from build123d import *

# Parameters (mm, degrees)
SKETCH_1_W          = 132
SKETCH_1_H          = 400
EXTRUDE_1_DEPTH     = 10
SKETCH_2_W          = 23
SKETCH_2_H          = 400
EXTRUDE_2_DEPTH     = 5
SKETCH_3_W          = 16
SKETCH_3_H          = 400
EXTRUDE_3_DEPTH     = 1
SKETCH_4_W          = 20
SKETCH_4_H          = 20
CUT_EXTRUDE_1_DEPTH = 11


with BuildPart() as part:
    # ｽｹｯﾁ1 → ﾎﾞｽ - 押し出し1 (new body)
    with BuildSketch(Plane.XY):
        with Locations((66, 200)):
            Rectangle(SKETCH_1_W, SKETCH_1_H)
    extrude(amount=EXTRUDE_1_DEPTH)

    # ｽｹｯﾁ2 → ﾎﾞｽ - 押し出し2 (add)
    with BuildSketch(Plane.XY.offset(10)):
        with Locations((11.5, 200)):
            Rectangle(SKETCH_2_W, SKETCH_2_H)
    extrude(amount=EXTRUDE_2_DEPTH)

    # ｽｹｯﾁ3 → ﾎﾞｽ - 押し出し3 (add)
    with BuildSketch(Plane.XY.offset(10)):
        with Locations((124, 200)):
            Rectangle(SKETCH_3_W, SKETCH_3_H)
    extrude(amount=EXTRUDE_3_DEPTH)

    # ｽｹｯﾁ4 → ｶｯﾄ - 押し出し1 (cut, through all)
    with BuildSketch(Plane.XY.offset(10)):
        with Locations((77.75, 200)):
            Rectangle(SKETCH_4_W, SKETCH_4_H)
    extrude(amount=-CUT_EXTRUDE_1_DEPTH, mode=Mode.SUBTRACT)


solid = part.part
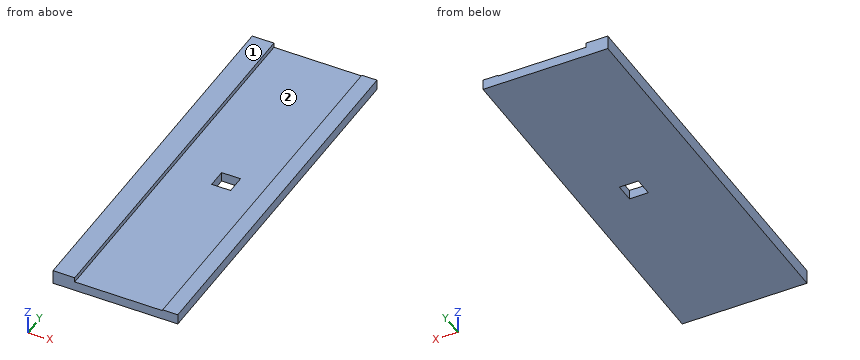
Here's how the part is built. I have some questions about the finished solid (model axes, mm). Face numbers are marked on the shaded views. Coordinates: 2 decimals unless noted, no trailing zeros. Write each loop counter-clockwise with the first axis right and the second up, starting at its lowest first coordinate (ties: lowest second). Pieces come first, ordered by that corner, then holes. Notation, with made-up numbers: (24, -1) - (39, -1) arc R16 ccw to (39, 26) - close; hole circle Ø3 at (-33, 86.5). An arc over 180 degrees is marked (long way). Use one line per item in the form item = value.
1) Suppose I cut it at A-A, the plane x = 73. Write out the boundary of the cut face in (y, z), plus the area to 3 significant figures.
Solved:
outline = (0, 0) - (190, 0) - (190, 10) - (0, 10) - close; (210, 0) - (400, 0) - (400, 10) - (210, 10) - close
area = 3,800 mm2
2) Thinking about a two-plate mould opening in X: for the marked faces 1 and 2, which applies, released by +X, released by -X, zero draft, split by the parting line, or undercut?
Solved:
face_1 = zero draft
face_2 = undercut
3) I need wall thicknesses on line 1 (Y direction, x = 73.5, z = 1.75); line 2 (X direction, y = 86, z = 10.75); line 3 (X direction, y = 104.5, z = 12). Which ranges of each line are inside material? Lowest first, please.
Solved:
line_1 = 0 to 190, 210 to 400
line_2 = 0 to 23, 116 to 132
line_3 = 0 to 23
4) Suppose I cut it at B-B, the plane y = 39.5. Write out the boundary of the cut face in (x, z), plus the area to 3 significant figures.
Solved:
outline = (0, 0) - (132, 0) - (132, 11) - (116, 11) - (116, 10) - (23, 10) - (23, 15) - (0, 15) - close
area = 1,450 mm2
5) I'm going to push flat-ended pins straight in: P1, Ø1, axis at x = 70, y = 354.5, coming from the +Z side; P2, Ø13, axis at x = 124.5, y = 150, coming from the +Z side. Where does each tip first touch, or does it pass through?
Solved:
P1 = 10
P2 = 11
6) Suppose I cut it at C-C, the plane x = 54.5. Write out the boundary of the cut face in (y, z), plus the area to 3 significant figures.
Solved:
outline = (0, 0) - (400, 0) - (400, 10) - (0, 10) - close
area = 4,000 mm2
7) Suppose I cut it at D-D, the plane x = 120. Write out the boundary of the cut face in (y, z).
Solved:
outline = (0, 0) - (400, 0) - (400, 11) - (0, 11) - close
